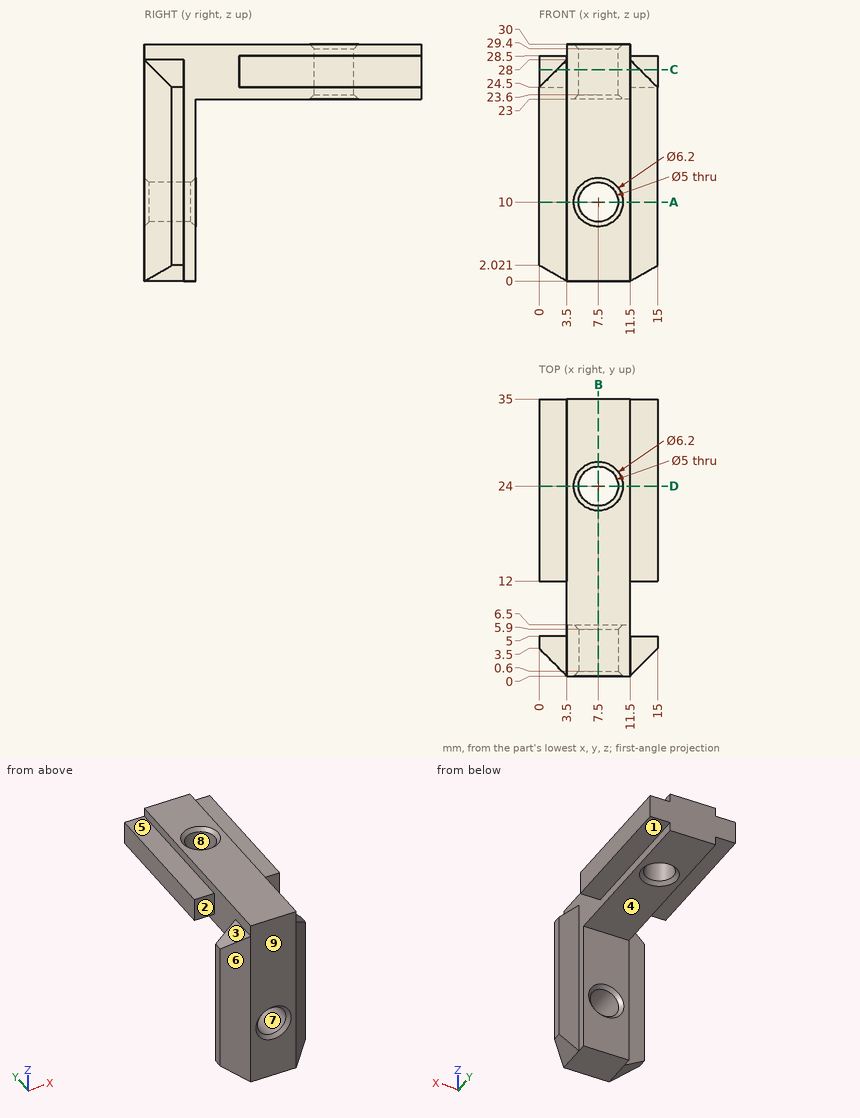
Geometry check sheet. Reference: drawing and pictorial views, mm from the part's lowest x, y, z. A direction names the side the tool comes from. Round coordinates to 2 decimals unless told otherwise and drop trailing zeros. Loops run counter-clockwise (first coordinate to the right, second up) from the corner with the lowest first, then second, coordinate; pieces in that order, holes last. Notation, with made-up numbers: (79, 85) - (112, 85) arc R29 ccw to (112, 118) - close; hole circle Ø3 at (28, -14). An arc over 180 degrees is marked (long way). Answer in a Markdown table with one row per item. Add a question column.
Q1. Section check A-A on z = 10. Enter the section's corners in (x, y).
Q2. Section check B-B on x = 7.5. Enter the section's corners in (y, z).
Q3. Release check for a two-part mould opening along X. For the marked faces 6, 7, 8 and 9 record: pulls with the +X half, pulls with the -X half, needs draft (parallel to the pull), parting line crosses it, or undercut.
Q4. Material ranges on line 1 (Y direction, x = 7.5, z = 25.9); line 2 (X direction, y = 24, z = 26.7); line 3 (Z direction, x = 2.5, y = 20), recorded low to high.
Q5. Section check D-D on y = 24. Enter the section's corners in (x, z), plus the area to 3 significant figures.
Q6. Section check C-C on z = 26.75. Enter the section's corners in (x, y), plus the area to 3 significant figures.
Q7. Tool access check on the marked faces 1, 2, 3, 4 and 5. Record the directions out of +Z, -Z, +X, -X, +Y, -Y that give a thin tool (end or side, any length) a straight path to the whole face; none if there is none.
Q8. Gauge pin test, flat ends, axial feed: pin 1 (2.5 mm diameter, centred on x = 7.5, z = 15, fed in from +Y); pin 2 (3 mm diameter, centred on x = 13.5, z = 25.5, fed in from -Y); pin 3 (1 mm diameter, centred on x = 12.5, y = 25.5, fed in from -Z). Record the tip position at first contact, or that the pin passes through.
Found:
| question | item | result |
|---|---|---|
| 1 | outline | (0, 3.5) - (3.5, 0) - (4.4, 0) - (5, 0.6) - (5, 5.9) - (4.4, 6.5) - (3.5, 6.5) - (3.5, 5) - (0, 5) - close; (10, 0.6) - (10.6, 0) - (11.5, 0) - (15, 3.5) - (15, 5) - (11.5, 5) - (11.5, 6.5) - (10.6, 6.5) - (10, 5.9) - close |
| 2 | outline | (0, 0) - (6.5, 0) - (6.5, 6.9) - (5.9, 7.5) - (0.6, 7.5) - (0, 6.9) - close; (0, 13.1) - (0.6, 12.5) - (5.9, 12.5) - (6.5, 13.1) - (6.5, 23) - (20.9, 23) - (21.5, 23.6) - (21.5, 29.4) - (20.9, 30) - (0, 30) - close; (26.5, 23.6) - (27.1, 23) - (35, 23) - (35, 30) - (27.1, 30) - (26.5, 29.4) - close |
| 3 | face 6 | pulls with the -X half |
| 3 | face 7 | undercut |
| 3 | face 8 | undercut |
| 3 | face 9 | needs draft |
| 4 | line 1 | y = 0 to 21.5, 26.5 to 35 |
| 4 | line 2 | x = 0 to 5, 10 to 15 |
| 4 | line 3 | z = 24.5 to 28.5 |
| 5 | outline | (0, 24.5) - (3.5, 24.5) - (3.5, 23) - (4.4, 23) - (5, 23.6) - (5, 29.4) - (4.4, 30) - (3.5, 30) - (3.5, 28.5) - (0, 28.5) - close; (10, 23.6) - (10.6, 23) - (11.5, 23) - (11.5, 24.5) - (15, 24.5) - (15, 28.5) - (11.5, 28.5) - (11.5, 30) - (10.6, 30) - (10, 29.4) - close |
| 5 | area | 48.3 mm² |
| 6 | outline | (0, 12) - (3.5, 12) - (3.5, 5) - (2.25, 5) - (2.25, 1.25) - (3.5, 0) - (11.5, 0) - (12.75, 1.25) - (12.75, 5) - (11.5, 5) - (11.5, 12) - (15, 12) - (15, 35) - (0, 35) - close; hole circle Ø5 at (7.5, 24) |
| 6 | area | 432 mm² |
| 7 | face 1 | -Z, +X, +Y |
| 7 | face 2 | +Z, -Z, -X |
| 7 | face 3 | +Z, -X, -Y |
| 7 | face 4 | -Z, +X, -X, +Y |
| 7 | face 5 | +Z, -X, +Y, -Y |
| 8 | pin 1 | stops at y = 6.5 |
| 8 | pin 2 | stops at y = 0.5 |
| 8 | pin 3 | stops at z = 24.5 |
